Work out the finished part from the listing and answer in its coordinate system (mm). Coordinates: 2 decimals unless noted, no trailing zeros. Loops run counter-clockwise (first coordinate to the right, second up) from the corner with the lowest first, then second, coordinate; pieces in that order, holes last. Notation, with made-up numbers: M 64.25,-16.5 L 110.25,-16.5 A30 cw 110.25,9.5 Z; hole C -7,68.25 d4. An arc over 180 degrees is marked long. Write each question's results on one line, items separated by ' | '.
```python
from build123d import *

# Parameters (mm, degrees)
F0_W     = 40
F0_H     = 7.5
F1_DEPTH = 3
F3_DEPTH = 10
F5_DEPTH = 3


with BuildPart() as f1:
    # F0 (on Top) → F1 (new body)
    with BuildSketch(Plane.XY):
        with Locations((-20, -3.75)):
            Rectangle(F0_W, F0_H)
    extrude(amount=F1_DEPTH)

    # F2 (on face) → F3 (cut)
    with BuildSketch(Plane.XZ.offset(7.5)):
        Polygon((-40, 3), (-40, 0), (-29.1941203177, 3), align=None)
    extrude(amount=-F3_DEPTH, mode=Mode.SUBTRACT)

    # F4 (on face) → F5 (cut)
    with BuildSketch(Plane.XY.offset(3)):
        with BuildLine():
            ThreePointArc((-3.75, 0), (-1.0983495706, -1.0983495706), (0, -3.75))
            Line((0, -3.75), (0, 0))
            Line((0, 0), (-3.75, 0))
        make_face()
        with BuildLine():
            Line((0, -7.5), (0, -3.75))
            ThreePointArc((0, -3.75), (-1.0983495706, -6.4016504294), (-3.75, -7.5))
            Line((-3.75, -7.5), (0, -7.5))
        make_face()
    extrude(amount=-F5_DEPTH, mode=Mode.SUBTRACT)


solid = f1.part
```
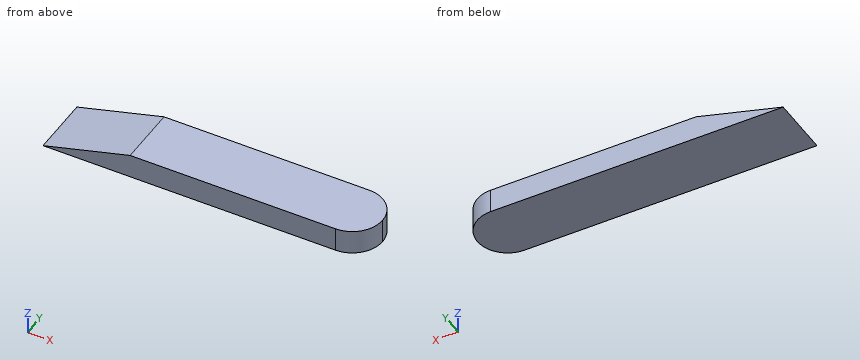
1) Find section D-D, the plane z = 2.35. Give the vertices of the cut face in (x, y).
Check result:
outline: M -31.54,-7.5 L -3.75,-7.5 A3.75 ccw -3.75,0 L -31.54,0 Z
2) Find section C-C, the plane x = -35. Give the vertices of the cut face in (y, z), and give its area (3 significant figures).
Check result:
outline: M -7.5,0 L 0,0 L 0,1.39 L -7.5,1.39 Z | area: 10.4 mm^2
3) Straight lines are drawn through the part: probe 1 along Z at (x, y) = (-30, -7); probe 2 along Z at (x, y) = (-36.5, -4.5); probe 3 along Y at (x, z) = (-3, 1.35). For each, find the intervals that lie inside material, in ascending order. Write a range as [from, to].
Check result:
probe 1: [0, 2.78] | probe 2: [0, 0.97] | probe 3: [-7.42, -0.08]
4) Find section A-A, the plane y = -1.5. Give the vertices of the cut face in (x, z).
Check result:
outline: M -40,0 L -0.75,0 L -0.75,3 L -29.19,3 Z
5) Find section B-B, the plane z = 0.7. Give the vertices of the cut face in (x, y).
Check result:
outline: M -37.48,-7.5 L -3.75,-7.5 A3.75 ccw -3.75,0 L -37.48,0 Z
